```python
from build123d import *

# Parameters (mm, degrees)
CROQUIS1_W              = 142
CROQUIS1_H              = 20.7
SALIENTE_EXTRUIR2_DEPTH = 3
CROQUIS6_R              = 1.5
CORTAR_EXTRUIR4_DEPTH   = 3
CROQUIS7_W              = 142
CROQUIS7_H              = 2
SALIENTE_EXTRUIR3_DEPTH = 9.7
CORTAR_EXTRUIR5_DEPTH   = 224
CROQUIS10_W             = 16.7
CROQUIS10_H             = 9.7
CORTAR_EXTRUIR6_DEPTH   = 10


with BuildPart() as part:
    # Croquis1 → Saliente-Extruir2 (new body)
    with BuildSketch(Plane(origin=(0, 0, 0), x_dir=(1, 0, 0), z_dir=(0, 1, 0))):
        Rectangle(CROQUIS1_W, CROQUIS1_H)
    extrude(amount=SALIENTE_EXTRUIR2_DEPTH)

    # Croquis6 → Cortar-Extruir4 (cut)
    with BuildSketch(Plane(origin=(0, 3, 0), x_dir=(1, 0, 0), z_dir=(0, 1, 0))):
        with Locations((-56, 0)):
            Circle(CROQUIS6_R)
        Circle(CROQUIS6_R)
        with Locations((56, 0)):
            Circle(CROQUIS6_R)
    extrude(amount=-CORTAR_EXTRUIR4_DEPTH, mode=Mode.SUBTRACT)

    # Croquis7 → Saliente-Extruir3 (add)
    with BuildSketch(Plane(origin=(0, 3, 0), x_dir=(1, 0, 0), z_dir=(0, 1, 0))):
        with Locations((0, 9.35)):
            Rectangle(CROQUIS7_W, CROQUIS7_H)
        with Locations((0, -9.35)):
            Rectangle(CROQUIS7_W, CROQUIS7_H)
    extrude(amount=SALIENTE_EXTRUIR3_DEPTH)

    # Croquis9 → Cortar-Extruir5 (cut)
    with BuildSketch(Plane.ZY.offset(71)):
        Polygon((-10.35, 2.7), (-9.85, 2.7), (-10.35, 1.2), align=None)
        Polygon((10.35, 2.7), (9.85, 2.7), (10.35, 1.2), align=None)
    extrude(amount=-CORTAR_EXTRUIR5_DEPTH, mode=Mode.SUBTRACT)

    # Croquis10 → Cortar-Extruir6 (cut)
    with BuildSketch(Plane.XY.offset(10.35)):
        with Locations((0, 7.85)):
            Rectangle(CROQUIS10_W, CROQUIS10_H)
    extrude(amount=-CORTAR_EXTRUIR6_DEPTH, mode=Mode.SUBTRACT)


solid = part.part
```
The listing builds one solid part. Answer for the finished solid, in the listing's coordinates (mm). A direction names the side the tool comes from. Round coordinates to 2 decimals unless told otherwise and drop trailing zeros. Loops run counter-clockwise (first coordinate to the right, second up) from the corner with the lowest first, then second, coordinate; pieces in that order, holes last. Notation, with made-up numbers: (76.25, -15) - (93.25, -15) arc R14 ccw to (93.25, 8) - close; hole circle Ø9 at (27.5, 11.25). An arc over 180 degrees is marked (long way). Return JSON: item names as keys, results as strings. Group by question number.
1. Which of the six approach directions +Z, -Z, +X, -X, +Y, -Y give full straight-line access (tool end or side, diameter ignored) to faces 4 (the flat face through (71, 2, 0)), 5 (the flat face through (-1, 8, -8.35))?
2. The part is cut by section D-D on x = 0. Determine the outline of the cut face in (y, z).
3. Consider probe 1 along X at (y, z) = (1.6, 0); probe 2 along Z at (x, y) = (-23.5, 6.75); probe 3 along X at (y, z) = (4.25, 9). Determine where each line is inside the solid, lowest interval first.
4. The mould has two halves that part along Z. Classify faces 1 (the cylindrical face through (-54.57, 1.52, -0.45)), 2 (the flat face through (-17, 8, 10.35)), 3 (the flat face through (-1, 0, -2)): pulls with the +Z half, pulls with the -Z half, needs draft (parallel to the pull), parting line crosses it, or undercut.
5. The part is cut by section C-C on y = 7. Determine the outline of the cut face in (x, z).
6. The part is cut by section A-A on z = 0. Determine the outline of the cut face in (x, y), then the cut area to 3 significant figures.
7. The part is cut by section B-B on x = -56. Determine the outline of the cut face in (y, z), then the cut area to 4 significant figures.
8. Each of these flat-tipped pins is pushed along its axis until it touches: P1, Ø2.5, axis at x = 56, z = 0, coming from the -Y side; P2, Ø3, axis at x = -52, z = -5, coming from the +Y side. Where does it stop, or does it pass through?
Resolved:
{
 "1": {"face 4": "+Z, -Z, +X, +Y, -Y", "face 5": "+X, -X, +Y"},
 "2": {"outline": "(0, -10.35) - (1.2, -10.35) - (2.7, -9.85) - (2.7, -10.35) - (12.7, -10.35) - (12.7, -8.35) - (3, -8.35) - (3, -1.5) - (0, -1.5) - close; (0, 1.5) - (3, 1.5) - (3, 10.35) - (2.7, 10.35) - (2.7, 9.85) - (1.2, 10.35) - (0, 10.35) - close"},
 "3": {"probe 1": "x = -71 to -57.5, -54.5 to -1.5, 1.5 to 54.5, 57.5 to 71", "probe 2": "z = -10.35 to -8.35, 8.35 to 10.35", "probe 3": "x = -71 to -8.35, 8.35 to 71"},
 "4": {"face 1": "undercut", "face 2": "pulls with the +Z half", "face 3": "needs draft"},
 "5": {"outline": "(-71, -10.35) - (71, -10.35) - (71, -8.35) - (-71, -8.35) - close; (-71, 8.35) - (-8.35, 8.35) - (-8.35, 10.35) - (-71, 10.35) - close; (8.35, 8.35) - (71, 8.35) - (71, 10.35) - (8.35, 10.35) - close"},
 "6": {"outline": "(-71, 0) - (-57.5, 0) - (-57.5, 3) - (-71, 3) - close; (-54.5, 0) - (-1.5, 0) - (-1.5, 3) - (-54.5, 3) - close; (1.5, 0) - (54.5, 0) - (54.5, 3) - (1.5, 3) - close; (57.5, 0) - (71, 0) - (71, 3) - (57.5, 3) - close", "area": "399 mm²"},
 "7": {"outline": "(0, -10.35) - (1.2, -10.35) - (2.7, -9.85) - (2.7, -10.35) - (12.7, -10.35) - (12.7, -8.35) - (3, -8.35) - (3, -1.5) - (0, -1.5) - close; (0, 1.5) - (3, 1.5) - (3, 8.35) - (12.7, 8.35) - (12.7, 10.35) - (2.7, 10.35) - (2.7, 9.85) - (1.2, 10.35) - (0, 10.35) - close", "area": "91.15 mm²"},
 "8": {"P1": "passes through", "P2": "stops at y = 3"}
}
